Drawing for the job (mm, zero at the part's lowest x, y, z). A direction names the side the tool comes from. Round coordinates to 2 decimals unless told otherwise and drop trailing zeros. Write each loop counter-clockwise with the first axis right and the second up, starting at its lowest first coordinate (ties: lowest second). Pieces come first, ordered by that corner, then holes.
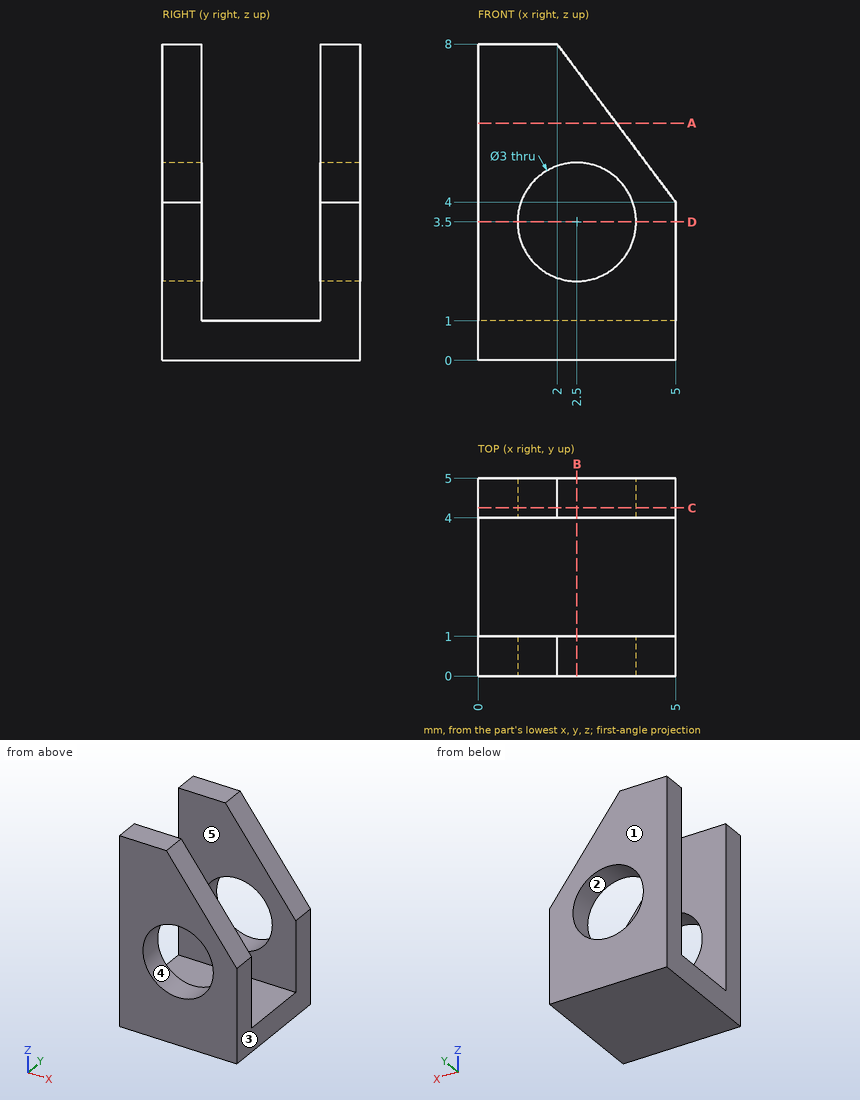
Q1. Tool access for the marked faces 4 and 5: list every direction of +Z, -Z, +X, -X, +Y, -Y with a clear straight run to the whole face (end or side of a thin tool).
Q2. Saw through at B-B, the plane x = 2.5. Write the cut outline in (y, z).
Q3. Drop flat-ended pins along their axis: P1, Ø3, axis at x = 3.5, y = 1, coming from the -Z side; P2, Ø1.5, axis at x = 3.5, y = 3, coming from the +Z side. Give the stop position or say it passes through.
Q4. Saw through at C-C, the plane y = 4.25. Write the cut outline in (x, z), and give its area (3 significant figures).
Q5. Wall check: line 1 (Y direction, x = 3.5, z = 4.75); line 2 (Z direction, x = 3.85, y = 1.9); line 3 (X direction, y = 0.6, z = 2.75). Give the ranges that are in metal, low to high.
Q6. Saw through at D-D, the plane z = 3.5. Write the cut outline in (x, y), and give its area (3 significant figures).
Q7. Two-plate mould, pull along X, no slides. Class the marked faces 1, 2 and 3: released by +X, released by -X, zero draft, split by the parting line, or undercut.
Q8. Saw through at A-A, the plane z = 6. Write the cut outline in (x, y), and give its area (3 significant figures).
Computed:
1. face 4: +Y, -Y
1. face 5: +Z, +X, -X
2. outline: (0, 0) - (5, 0) - (5, 2) - (4, 2) - (4, 1) - (1, 1) - (1, 2) - (0, 2) - close; (0, 5) - (1, 5) - (1, 7.33) - (0, 7.33) - close; (4, 5) - (5, 5) - (5, 7.33) - (4, 7.33) - close
3. P1: stops at z = 0
3. P2: stops at z = 1
4. outline: (0, 0) - (5, 0) - (5, 4) - (2, 8) - (0, 8) - close; hole circle Ø3 at (2.5, 3.5)
4. area: 26.9 mm2
5. line 1: y = 0 to 1, 4 to 5
5. line 2: z = 0 to 1
5. line 3: x = 0 to 1.2, 3.8 to 5
6. outline: (0, 0) - (1, 0) - (1, 1) - (0, 1) - close; (0, 4) - (1, 4) - (1, 5) - (0, 5) - close; (4, 0) - (5, 0) - (5, 1) - (4, 1) - close; (4, 4) - (5, 4) - (5, 5) - (4, 5) - close
6. area: 4.00 mm2
7. face 1: zero draft
7. face 2: undercut
7. face 3: released by +X
8. outline: (0, 0) - (3.5, 0) - (3.5, 1) - (0, 1) - close; (0, 4) - (3.5, 4) - (3.5, 5) - (0, 5) - close
8. area: 7.00 mm2
